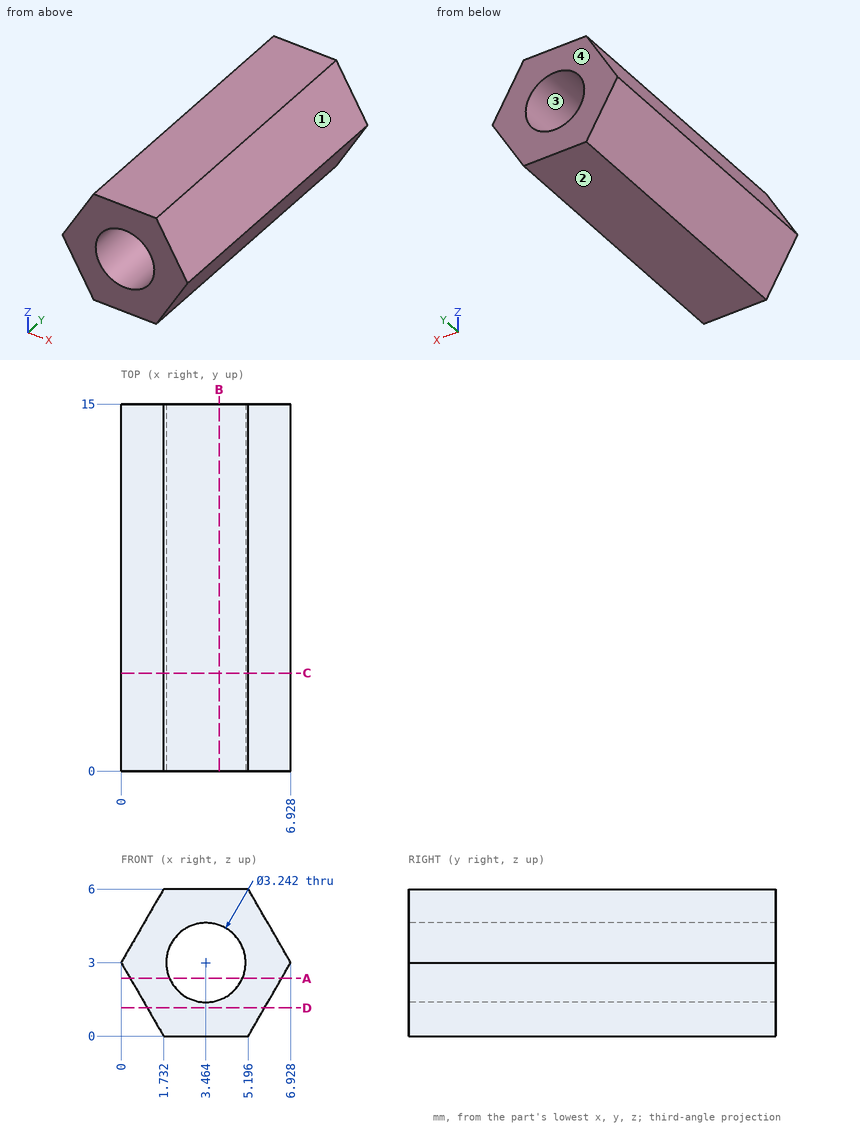
Answer from the drawing. Dimensions are ordinates in mm from the lowest x, y and z of the part. Coordinates: 2 decimals unless noted, no trailing zeros. Write each loop counter-clockwise with the first axis right and the second up, starting at its lowest first coordinate (ties: lowest second). Pieces come first, ordered by that corner, then holes. Notation, with made-up numbers: (74.25, -33) - (114.25, -33) arc R19 cw to (114.25, -24) - close; hole circle Ø5 at (77.5, 81.25). An arc over 180 degrees is marked (long way). Return JSON: item names as keys, results as strings.
1. The part is cut by section C-C on y = 4. Determine the outline of the cut face in (x, z), then the cut area to 3 significant figures.
Final values:
{"outline": "(0, 3) - (1.73, 0) - (5.2, 0) - (6.93, 3) - (5.2, 6) - (1.73, 6) - close; hole circle Ø3.24 at (3.46, 3)", "area": "22.9 mm^2"}
2. Consider line 1 along X through (y, z) = (3.25, 3.55); line 2 along Z through (x, y) = (2.75, 13.25) (1 decimal); line 3 along X through (y, z) = (10.25, 1.65). Determine where each line is inside the solid, lowest interval first.
Final values:
{"line 1": "0.32 to 1.94, 4.99 to 6.61", "line 2": "0 to 1.5, 4.5 to 6", "line 3": "0.78 to 2.57, 4.36 to 6.15"}
3. For a pull along Z with two mould halves and no side action, classify the marked faces 1, 2, 3 and 4 as +Z half, -Z half, draft (parallel to the pull), parting line (faces both ways), or undercut.
Final values:
{"face 1": "+Z half", "face 2": "-Z half", "face 3": "undercut", "face 4": "draft"}
4. Each of these flat-tipped pins is pushed along its axis until it touches: pin 1 Ø3 at (x, z) = (3.46, 3) entering from +Y; pin 2 Ø3 at (x, z) = (4, 1) entering from -Y; pin 3 Ø2 at (y, z) = (13, 5) entering from -X; pin 4 Ø1 at (y, z) = (6.5, 2) entering from +X. Where does it stop, or does it pass through?
Final values:
{"pin 1": "through", "pin 2": "y = 0", "pin 3": "x = 0.58", "pin 4": "x = 6.64"}
5. The part is cut by section A-A on z = 2.35. Determine the outline of the cut face in (x, y) (1 decimal), then the cut area to 3 significant figures.
Final values:
{"outline": "(0.4, 0) - (2, 0) - (2, 15) - (0.4, 15) - close; (4.9, 0) - (6.6, 0) - (6.6, 15) - (4.9, 15) - close", "area": "48.1 mm^2"}
6. The part is cut by section B-B on x = 4. Determine the outline of the cut face in (y, z).
Final values:
{"outline": "(0, 0) - (15, 0) - (15, 1.47) - (0, 1.47) - close; (0, 4.53) - (15, 4.53) - (15, 6) - (0, 6) - close"}
7. The part is cut by section D-D on z = 1.15. Determine the outline of the cut face in (x, y), then the cut area to 3 significant figures.
Final values:
{"outline": "(1.07, 0) - (5.86, 0) - (5.86, 15) - (1.07, 15) - close", "area": "71.9 mm^2"}
